Verification items for the finished model (mm, model axes). A direction names the side the tool comes from. Coordinates: 2 decimals unless noted, no trailing zeros. Write each loop counter-clockwise with the first axis right and the second up, starting at its lowest first coordinate (ties: lowest second). Pieces come first, ordered by that corner, then holes. Notation, with made-up numbers: (51.25, 4) -> (97.25, 4) arc R11 ccw to (97.25, 9) -> close; hole circle Ø4 at (24, -15.75). An arc over 180 degrees is marked (long way). Answer in a Markdown table with one row per item.
Autodesk Inventor part; units mm, degrees
ref_plane "rod_cp_XY" through (0, 0, 0) normal (1, 0, 0) x (0, 0, -1)
ref_plane "rod_cp_YZ" through (0, 0, 0) normal (0, 0, -1) x (0, 1, 0)
ref_plane "rod_cp_ZX" through (0, 0, 0) normal (0, 1, 0) x (1, 0, 0)
sketch "Sketch_1" plane through (0, 0, 0) normal (0, 0, 1) x (1, 0, 0)
  line L0 (290.5252, 0) -> (0, 0)
  line L1 (0, 0) -> (0, 3.175)
  line L2 (0, 3.175) -> (269.0876, 3.175)
  line L3 (269.0876, 3.175) -> (269.0876, 9.6203)
  line L4 (269.0876, 9.6203) -> (290.5252, 9.6203)
  line L5 (290.5252, 9.6203) -> (290.5252, 0)
  line L6 (290.5252, 0) -> (0, 0)
revolve "Revolution1" add sketch "Sketch_1" angle 360 about axis through (290.5252, 0, 0) along (1, 0, 0)
sketch "Sketch_3" plane through (0, 0, 0) normal (0, 0, 1) x (1, 0, 0)
  line L0 (0, 0) -> (-12.7, 0)
  line L1 (-12.7, 0) -> (-12.7, 2.634)
  line L2 (-12.7, 2.634) -> (-12.159, 3.175)
  line L3 (-12.159, 3.175) -> (0, 3.175)
  line L4 (0, 3.175) -> (0, 0)
  line L5 (0, 0) -> (-12.7, 0)
revolve "Revolution2" add sketch "Sketch_3" angle 360 about axis through (0, 0, 0) along (1, 0, 0)
thread "Thread1"
sketch "Sketch_30" plane through (0, 0, 0) normal (0, 0, 1) x (1, 0, 0)
  line L0 (0, 0) -> (-0.254, 0)
  line L1 (-0.254, 3.429) -> (-0.254, 2.921)
  line L2 (-0.254, 2.921) -> (0, 2.921)
  line L3 (0, 2.921) -> (0, 3.429)
  line L4 (0, 3.429) -> (-0.254, 3.429)
revolve "Revolution3" cut sketch "Sketch_30" angle 360 about axis through (0, 0, 0) along (1, 0, 0)
ref_plane "rod_cp_XY" through (0, 0, 0) normal (1, 0, 0) x (0, 0, -1)
ref_plane "rod_cp_YZ" through (0, 0, 0) normal (0, 0, -1) x (0, 1, 0)
ref_plane "rod_cp_ZX" through (0, 0, 0) normal (0, 1, 0) x (1, 0, 0)
ref_plane "to_rod_clevis_XY" through (-12.7, 0, 0) normal (1, 0, 0) x (0, 0, -1)
ref_plane "to_rod_clevis_YZ" through (-12.7, 0, 0) normal (0, 0, -1) x (0, 1, 0)
ref_plane "to_rod_clevis_ZX" through (-12.7, 0, 0) normal (0, 1, 0) x (1, 0, 0)
ref_plane "rl2_XY" through (0, 0, 0) normal (1, 0, 0) x (0, 0, -1)
ref_plane "rl2_YZ" through (0, 0, 0) normal (0, 0, -1) x (0, 1, 0)
ref_plane "rl2_ZX" through (0, 0, 0) normal (0, 1, 0) x (1, 0, 0)
ref_plane "rl1_XY" through (-12.7, 0, 0) normal (1, 0, 0) x (0, 0, -1)
ref_plane "rl1_YZ" through (-12.7, 0, 0) normal (0, 0, -1) x (0, 1, 0)
ref_plane "rl1_ZX" through (-12.7, 0, 0) normal (0, 1, 0) x (1, 0, 0)
ref_plane "thd1_XY" through (-12.7, 3.175, 0) normal (1, 0, 0) x (0, 0, -1)
ref_plane "thd1_YZ" through (-12.7, 3.175, 0) normal (0, 0, -1) x (0, 1, 0)
ref_plane "thd1_ZX" through (-12.7, 3.175, 0) normal (0, 1, 0) x (1, 0, 0)
ref_plane "thd2_XY" through (-12.7, -3.175, 0) normal (1, 0, 0) x (0, 0, -1)
ref_plane "thd2_YZ" through (-12.7, -3.175, 0) normal (0, 0, -1) x (0, 1, 0)
ref_plane "thd2_ZX" through (-12.7, -3.175, 0) normal (0, 1, 0) x (1, 0, 0)
ref_plane "dia1_XY" through (0, 3.175, 0) normal (1, 0, 0) x (0, 0, -1)
ref_plane "dia1_YZ" through (0, 3.175, 0) normal (0, 0, -1) x (0, 1, 0)
ref_plane "dia1_ZX" through (0, 3.175, 0) normal (0, 1, 0) x (1, 0, 0)
ref_plane "dia2_XY" through (0, -3.175, 0) normal (1, 0, 0) x (0, 0, -1)
ref_plane "dia2_YZ" through (0, -3.175, 0) normal (0, 0, -1) x (0, 1, 0)
ref_plane "dia2_ZX" through (0, -3.175, 0) normal (0, 1, 0) x (1, 0, 0)
ref_plane "hh1_XY" through (320.6496, 0, 0) normal (0, 0, 1) x (1, 0, 0)
ref_plane "hh1_YZ" through (320.6496, 0, 0) normal (1, 0, 0) x (0, 1, 0)
ref_plane "hh1_ZX" through (320.6496, 0, 0) normal (0, 1, 0) x (0, 0, 1)
ref_plane "hh2_XY" through (327.0504, 0, 0) normal (0, 0, 1) x (1, 0, 0)
ref_plane "hh2_YZ" through (327.0504, 0, 0) normal (1, 0, 0) x (0, 1, 0)
ref_plane "hh2_ZX" through (327.0504, 0, 0) normal (0, 1, 0) x (0, 0, 1)
ref_plane "dia12_XY" through (0, 0, 10.9537) normal (1, 0, 0) x (0, 0, -1)
ref_plane "dia12_YZ" through (0, 0, 10.9537) normal (0, 0, -1) x (0, 1, 0)
ref_plane "dia12_ZX" through (0, 0, 10.9537) normal (0, 1, 0) x (1, 0, 0)
ref_plane "dia22_XY" through (0, 0, -10.9537) normal (1, 0, 0) x (0, 0, -1)
ref_plane "dia22_YZ" through (0, 0, -10.9537) normal (0, 0, -1) x (0, 1, 0)
ref_plane "dia22_ZX" through (0, 0, -10.9537) normal (0, 1, 0) x (1, 0, 0)
properties part number "049-DXP0_rod"
1. Go/stop test with flat-tipped pins: pin 1 (8 mm diameter, centred on x = 155.5, z = -6, fed in from -Y); pin 2 (6 mm diameter, centred on x = 112, z = 2.5, fed in from -Y) (3 decimals); pin 3 (4 mm diameter, centred on x = 35.5, y = 0, fed in from +Z) (3 decimals). Record where each tip stops, or that it passes through.
Findings below:
| item | result |
|---|---|
| pin 1 | stops at y = -2.47 |
| pin 2 | stops at y = -3.175 |
| pin 3 | stops at z = 3.175 |
2. Material ranges on probe 1 along Z at (x, y) = (244.5, -0.5); probe 2 along X at (y, z) = (3.5, -1.5); probe 3 along Z at (x, y) = (144, 1.75), recorded low to high. Write a range as from..to.
Findings below:
| item | result |
|---|---|
| probe 1 | z = -3.14..3.14 |
| probe 2 | x = 269.09..290.53 |
| probe 3 | z = -2.65..2.65 |
3. Access from +Z, -Z, +X, -X, +Y, -Y to the whole of each face (thin tool, end or side, straight path). Record for faces 1 (the face through (279.96, -2.09, -9.39)), 2 (the face through (269.088, 4, 0)).
Findings below:
| item | result |
|---|---|
| face 1 | +X, -X |
| face 2 | -X |
4. Sectioned sample at A-A, the plane z = 0. Record the cut outline in (x, y) (3 decimals).
Findings below:
| item | result |
|---|---|
| outline | (-12.7, -2.634) -> (-12.159, -3.175) -> (-0.254, -3.175) -> (-0.254, -2.921) -> (0, -2.921) -> (0, -3.175) -> (269.088, -3.175) -> (269.088, -9.62) -> (290.525, -9.62) -> (290.525, 9.62) -> (269.088, 9.62) -> (269.088, 3.175) -> (0, 3.175) -> (0, 2.921) -> (-0.254, 2.921) -> (-0.254, 3.175) -> (-12.159, 3.175) -> (-12.7, 2.634) -> close |
